Read the model definition and answer for the solid it produces. Units are mm, in the model's axes. Face numbers are marked on the shaded views. Give positions to 0.01 mm unless a question says otherwise; leave off trailing zeros. Write each loop counter-clockwise with the first axis right and the second up, starting at its lowest first coordinate (ties: lowest second). Pieces come first, ordered by that corner, then holes. Notation, with made-up numbers: M 38.5,-14 L 55.5,-14 A23 ccw 55.5,-5 Z; hole C 86,-18 d1. An arc over 180 degrees is marked long. Use a Markdown table: item, result. Add a question column.
Item 1: A cutting plane is placed at C-C on y = -7. Determine the outline of the cut face in (x, z), then the cut area to 3 significant figures.
Item 2: The mould has two halves that part along Z. Classify the marked faces 1, 2 and 3: pulls with the +Z half, pulls with the -Z half, needs draft (parallel to the pull), parting line crosses it, or undercut.
Item 3: A cutting plane is placed at B-B on x = 5. Determine the outline of the cut face in (y, z), then the cut area to 3 significant figures.
Item 4: A cutting plane is placed at D-D on z = -8.5. Determine the outline of the cut face in (x, y), then the cut area to 3 significant figures.
Item 5: Consider probe 1 along Z at (x, y) = (0, -1.6); probe 2 along Y at (x, z) = (3.5, 35.5); probe 3 along X at (y, z) = (-5.5, 23). Determine where each line is inside the solid, lowest interval first. Write a range as [from, to].
Item 6: A cutting plane is placed at A-A on y = -0.75. Determine the outline of the cut face in (x, z), then the cut area to 3 significant figures.
Item 7: Given P1, Ø1.5, axis at x = 8.5, y = -3, coming from the +Z side; P2, Ø4, axis at y = -2.5, z = 40, coming from the +X side; P3, Ø4, axis at y = -1.5, z = 41, coming from the -X side, each flat-ended and moving along its own axis, determine where each tip first touches the part or whether it passes through.
from build123d import *

# Parameters (mm, degrees)
F0_R       = 2.5
F1_DEPTH   = 5
F2_SIZE    = 7
F3_DEPTH   = 10
F4_R       = 5
F5_DEPTH   = 9
F6_SIZE2   = 3.9
F6_SIZE    = 4.4864367882
F6_2_SIZE2 = 3.9
F6_2_SIZE  = 4.4864367882
F6_3_SIZE2 = 3.9
F6_3_SIZE  = 4.4864367882


# Not quite as in the source:
# - a feature names something its author has since deleted; it is built from what else it names


with BuildPart() as f1:
    # F0 (on Front) → F1 (new body)
    with BuildSketch(Plane.XZ):
        Polygon((17.5, -37.5), (17.5, 37.5), (7.5, 37.5), (0, 37.5), (-7.5, 37.5), (-17.5, 37.5), (-17.5, -37.5), align=None)
        Polygon((0, -11.1), (-15, -1.1), (15, -1.1), align=None, mode=Mode.SUBTRACT)
        Polygon((0, 3.2), (-15, 13.2), (15, 13.2), align=None, mode=Mode.SUBTRACT)
        Polygon((0, 17.5), (-15, 27.5), (15, 27.5), align=None, mode=Mode.SUBTRACT)
        Polygon((0, 37.5), (7.5, 37.5), (7.5, 47.5), (0, 47.5), (-7.5, 47.5), (-7.5, 37.5), align=None)
        with Locations((0, 42.5)):
            Circle(F0_R, mode=Mode.SUBTRACT)
    extrude(amount=F1_DEPTH)

    # F2
    f2_edges = [f1.edges().sort_by_distance(p)[0] for p in [
        (-17.5, -2.5, 37.5),
        (17.5, -2.5, 37.5),
        (-17.5, -2.5, -37.5),
        (17.5, -2.5, -37.5),
    ]]
    chamfer(f2_edges, length=F2_SIZE)

    # F0 (on Front) → F3 (cut)
    with BuildSketch(Plane.XZ):
        with Locations((0, 42.5)):
            Circle(F0_R)
    extrude(amount=-F3_DEPTH, mode=Mode.SUBTRACT)

    # F4
    f4_edges = [f1.edges().sort_by_distance(p)[0] for p in [
        (-7.5, -2.5, 47.5),
        (7.5, -2.5, 47.5),
    ]]
    fillet(f4_edges, radius=F4_R)

    # F0 (on Front) → F5 (join)
    with BuildSketch(Plane.XZ):
        Polygon((15, 27.5), (-15, 27.5), (0, 17.5), align=None)
        Polygon((15, 13.2), (-15, 13.2), (0, 3.2), align=None)
        Polygon((15, -1.1), (-15, -1.1), (0, -11.1), align=None)
    extrude(amount=F5_DEPTH)

    # F6
    f6_edges = [f1.edges().sort_by_distance(p)[0] for p in [
        (0, -9, -1.1),
        (-7.5, -9, -6.1),
        (7.5, -9, -6.1),
    ]]
    f6_side = f1.faces().sort_by_distance((0, -9, -4.433333))[0]
    chamfer(f6_edges, length=F6_SIZE, length2=F6_SIZE2, reference=f6_side)

    # F6#2
    f6_2_edges = [f1.edges().sort_by_distance(p)[0] for p in [
        (0, -9, 13.2),
        (-7.5, -9, 8.2),
        (7.5, -9, 8.2),
    ]]
    f6_2_side = f1.faces().sort_by_distance((0, -9, 9.866667))[0]
    chamfer(f6_2_edges, length=F6_2_SIZE, length2=F6_2_SIZE2, reference=f6_2_side)

    # F6#3
    f6_3_edges = [f1.edges().sort_by_distance(p)[0] for p in [
        (0, -9, 27.5),
        (-7.5, -9, 22.5),
        (7.5, -9, 22.5),
    ]]
    f6_3_side = f1.faces().sort_by_distance((0, -9, 24.166667))[0]
    chamfer(f6_3_edges, length=F6_3_SIZE, length2=F6_3_SIZE2, reference=f6_3_side)


solid = f1.part
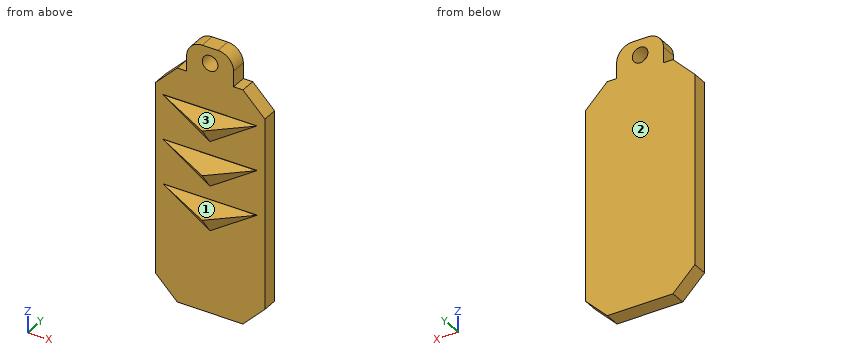
Filled in:
| question | item | result |
|---|---|---|
| 1 | outline | M -7.78,-3.29 L 0,-8.47 L 7.78,-3.29 Z; M -7.78,11.01 L 0,5.83 L 7.78,11.01 Z; M -7.78,25.31 L 0,20.13 L 7.78,25.31 Z |
| 1 | area | 121 mm² |
| 2 | face 1 | undercut |
| 2 | face 2 | needs draft |
| 2 | face 3 | pulls with the +Z half |
| 3 | outline | M -7.73,-4.13 L -5.1,-7.77 L -5,-7.77 L -5,-37.5 L 0,-37.5 L 0,46.83 L -5,46.83 L -5,27.5 L -5.1,27.5 L -7.73,24.47 L -5.1,20.83 L -5,20.83 L -5,13.2 L -5.1,13.2 L -7.73,10.17 L -5.1,6.53 L -5,6.53 L -5,-1.1 L -5.1,-1.1 Z |
| 3 | area | 450 mm² |
| 4 | outline | M -17.5,-5 L -3.9,-5 L -3.9,-5.1 L 0,-6.98 L 3.9,-5.1 L 3.9,-5 L 17.5,-5 L 17.5,0 L -17.5,0 Z |
| 4 | area | 183 mm² |
| 5 | probe 1 | [-37.5, 40], [45, 47.5] |
| 5 | probe 2 | [-5, 0] |
| 5 | probe 3 | [-7.42, 7.42] |
| 6 | outline | M -17.5,-30.5 L -10.5,-37.5 L 10.5,-37.5 L 17.5,-30.5 L 17.5,30.5 L 10.5,37.5 L 7.5,37.5 L 7.5,42.5 A5 ccw 2.5,47.5 L -2.5,47.5 A5 ccw -7.5,42.5 L -7.5,37.5 L -10.5,37.5 L -17.5,30.5 Z; hole C 0,42.5 d5 |
| 6 | area | 2,650 mm² |
| 7 | P1 | z = 37.5 |
| 7 | P2 | x = 7.5 |
| 7 | P3 | x = -7.5 |
